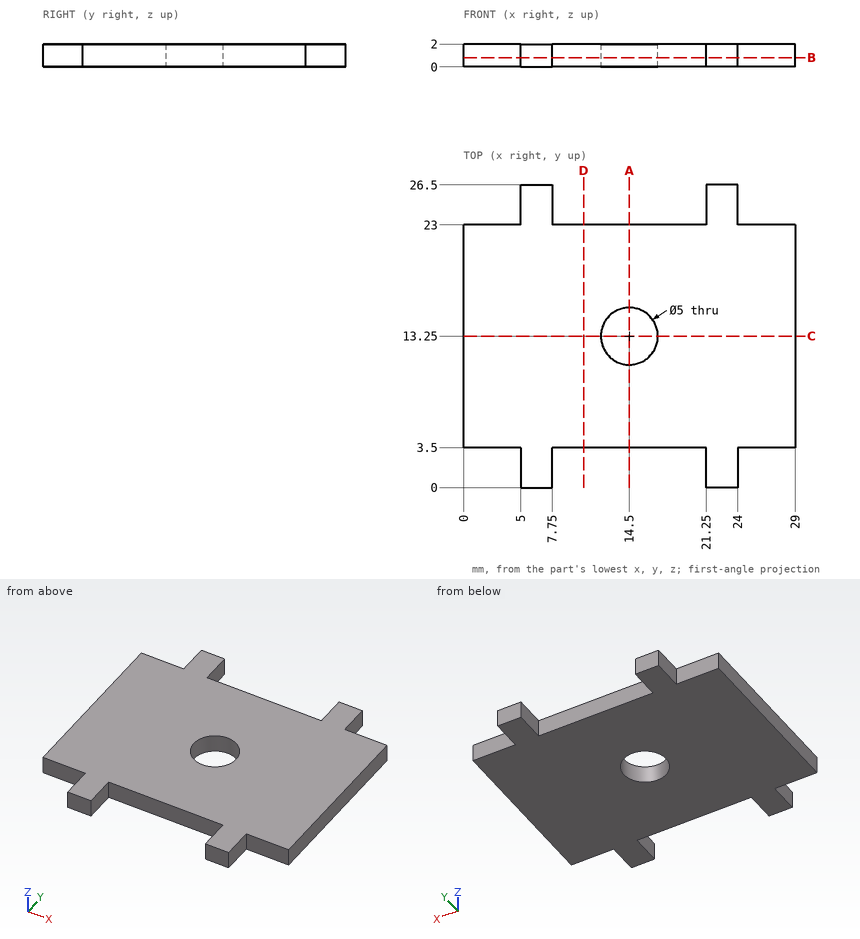
Design review of the part shown in the three views and the two pictorial views. Dimensions are in mm from the part's minimum x, y and z. Round coordinates to 2 decimals unless told otherwise and drop trailing zeros. Write each loop counter-clockwise with the first axis right and the second up, starting at its lowest first coordinate (ties: lowest second). Pieces come first, ordered by that corner, then holes. Notation, with made-up numbers: (-12.5, 9.25) - (-0.5, 9.25) arc R26 ccw to (-0.5, 42.25) - close; hole circle Ø4 at (-38, 19). An arc over 180 degrees is marked (long way). Answer as CSV lines item,"result". Start each with the question number.
(1) Add section A-A, the plane x = 14.5. State the section outline as (y, z) points.
(2) For line 1 (X direction, y = 23.5, z = 1.8); line 2 (Y direction, x = 14.5, z = 1); line 3 (Y direction, x = 27.5, z = 1.65), list the stretches that pass through material, from the lowest coordinate up.
(3) Add section D-D, the plane x = 10.5. State the section outline as (y, z) points, plus the area to 3 significant figures.
(4) Add section B-B, the plane z = 0.8. State the section outline as (x, y) points.
(5) For pin 1 (2 mm diameter, centred on x = 11, y = 12, fed in from -Z); pin 2 (1 mm diameter, centred on y = 24, z = 1.5, fed in from -X); pin 3 (1 mm diameter, centred on x = 14.5, z = 0.5, fed in from -Y); pin 4 (1 mm diameter, centred on y = 2, z = 0.5, fed in from +X), all flat-tipped, find the tip position at first contact; note any pin that passes through.
(6) Add section C-C, the plane y = 13.25. State the section outline as (x, z) points, plus the area to 3 significant figures.
From the geometry:
1,outline,"(3.5, 0) - (10.75, 0) - (10.75, 2) - (3.5, 2) - close; (15.75, 0) - (23, 0) - (23, 2) - (15.75, 2) - close"
2,line 1,"x = 5 to 7.75, 21.25 to 24"
2,line 2,"y = 3.5 to 10.75, 15.75 to 23"
2,line 3,"y = 3.5 to 23"
3,outline,"(3.5, 0) - (23, 0) - (23, 2) - (3.5, 2) - close"
3,area,"39.0 mm²"
4,outline,"(0, 3.5) - (5, 3.5) - (5, 0) - (7.75, 0) - (7.75, 3.5) - (21.25, 3.5) - (21.25, 0) - (24, 0) - (24, 3.5) - (29, 3.5) - (29, 23) - (24, 23) - (24, 26.5) - (21.25, 26.5) - (21.25, 23) - (7.75, 23) - (7.75, 26.5) - (5, 26.5) - (5, 23) - (0, 23) - close; hole circle Ø5 at (14.5, 13.25)"
5,pin 1,"stops at z = 0"
5,pin 2,"stops at x = 5"
5,pin 3,"stops at y = 3.5"
5,pin 4,"stops at x = 24"
6,outline,"(0, 0) - (12, 0) - (12, 2) - (0, 2) - close; (17, 0) - (29, 0) - (29, 2) - (17, 2) - close"
6,area,"48.0 mm²"
